Source: three-view drawing plus pictorial views. Frame: mm from the lowest corner of the part. A direction names the side the tool comes from. Give positions to 0.01 mm unless a question says otherwise; leave off trailing zeros. Loops run counter-clockwise (first coordinate to the right, second up) from the corner with the lowest first, then second, coordinate; pieces in that order, holes last. Notation, with made-up numbers: M -36,62 L 6,62 A28 cw 6,87 Z; hole C 73.25,39.5 d10. An arc over 180 degrees is marked long. Write item = value, one per line.
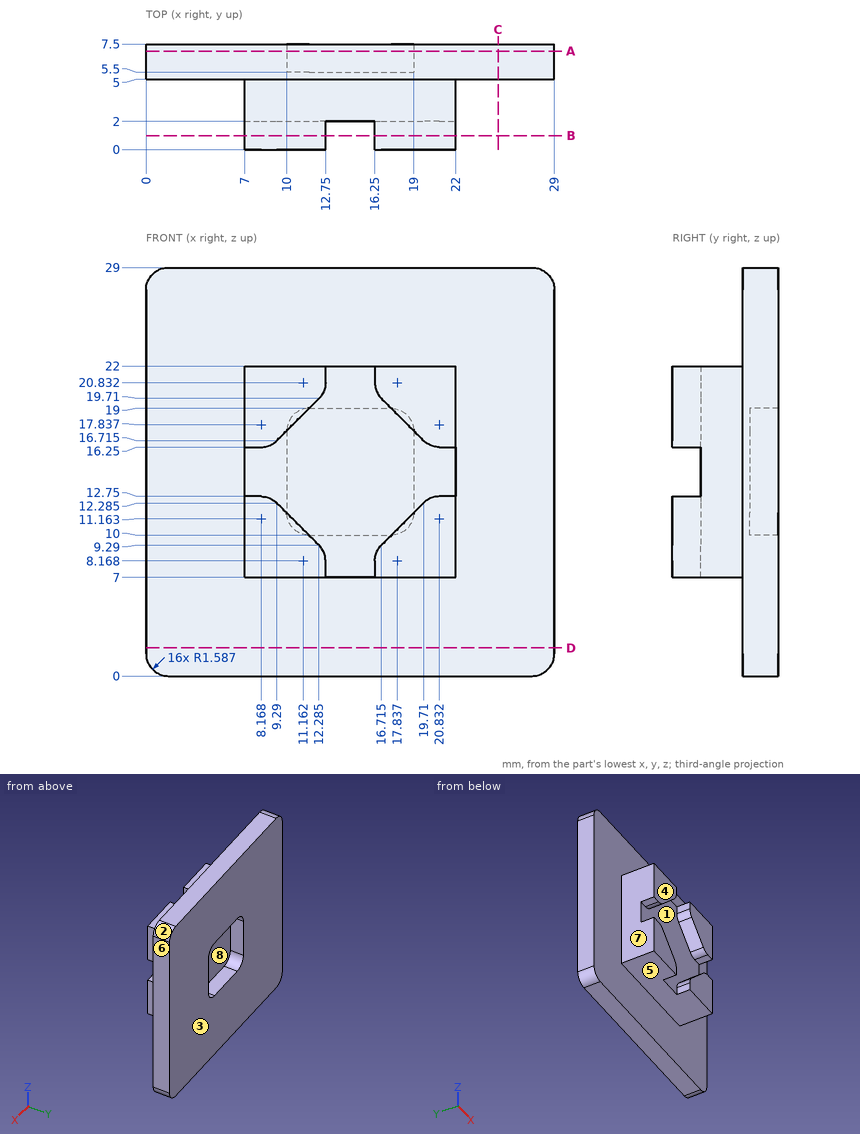
1. First-contact query: pin 1 Ø0.6 at (x, y) = (7.5, 1) entering from +Z; pin 2 Ø4 at (x, z) = (16, 16.5) entering from -Y; pin 3 Ø4 at (y, z) = (2, 16.5) entering from -X. Flat tips, straight axial feed; report the tip coordinate or a pass-through.
Derived:
pin_1 = 22
pin_2 = 2
pin_3 = 7
2. Reachability of the marked faces 4, 5, 6, 7 and 8 from +Z, -Z, +X, -X, +Y, -Y: full face, straight path, thin tool, end or side. Return the list, or none.
Derived:
face_4 = +Z, -Z, +X, -X, -Y
face_5 = -Z, +X, -X, -Y
face_6 = +Z, -Z, +X, +Y, -Y
face_7 = +Z, -Z, -X, -Y
face_8 = +Y
3. Cut plane D-D, the plane z = 2. Return the cut outline in (x, y).
Derived:
outline = M 0,5 L 29,5 L 29,7.5 L 0,7.5 Z
4. Pull-direction query (X, two-part tool) for the marked faces 1, 2 and 3; classes: +X half, -X half, draft (parallel to the pull), parting line (faces both ways), or undercut.
Derived:
face_1 = undercut
face_2 = +X half
face_3 = draft
5. Cut plane B-B, the plane y = 1. Count the separate pieces of the cut face and the enclosed holes in it, then the cut area to 3 significant figures.
Derived:
separate_pieces = 4
enclosed_holes = 0
area = 101 mm²
6. Cut plane A-A, the plane y = 7. Return the cut outline in (x, z) (1 decimal), then the cut area to 3 significant figures.
Derived:
outline = M 0,1.6 A1.6 ccw 1.6,0 L 27.4,0 A1.6 ccw 29,1.6 L 29,27.4 A1.6 ccw 27.4,29 L 1.6,29 A1.6 ccw 0,27.4 Z; hole M 10,11.6 A1.6 ccw 11.6,10 L 17.4,10 A1.6 ccw 19,11.6 L 19,17.4 A1.6 ccw 17.4,19 L 11.6,19 A1.6 ccw 10,17.4 Z
area = 760 mm²
7. Cut plane C-C, the plane x = 25. Return the cut outline in (y, z).
Derived:
outline = M 5,0 L 7.5,0 L 7.5,29 L 5,29 Z
8. Material intervals for probe 1 along Z at (x, y) = (16, 6); probe 2 along X at (y, z) = (2.25, 12.5); probe 3 along Y at (x, z) = (18.25, 17.5), sorted ascending. Write a range as from..to.
Derived:
probe_1 = 0..10, 19..29
probe_2 = 7..22
probe_3 = 2..5.5
